Check sheet for the modelled part. Datum: model origin and axes. Units: mm. Face numbers are marked on the shaded views. A direction names the side the tool comes from. Give positions to 0.01 mm unless a question says otherwise; leave off trailing zeros. Order: outer loops, then holes, each group sorted by start corner. A loop starts at its lowest first (then second) coordinate and runs counter-clockwise, first axis right, second up.
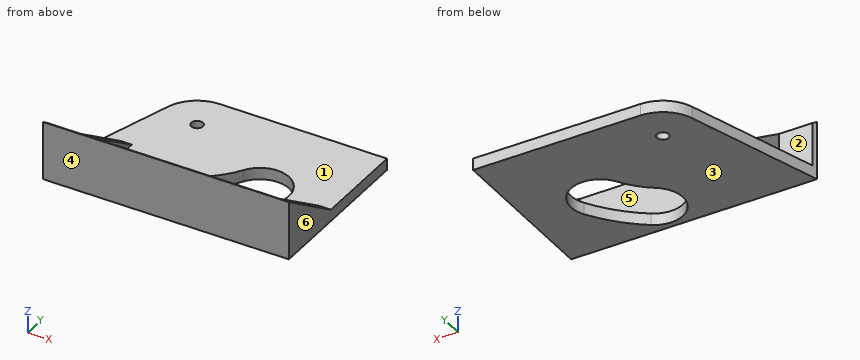
```python
from build123d import *

# Parameters (mm, degrees)
SKETCH1_W           = 120
SKETCH1_H           = 100
BOSS_EXTRUDE1_DEPTH = 5
SKETCH2_R           = 2.5
CUT_EXTRUDE1_DEPTH  = 6
SKETCH3_W           = 120
SKETCH3_H           = 2
BOSS_EXTRUDE2_DEPTH = 20
CUT_EXTRUDE2_DEPTH  = 26
CUT_EXTRUDE3_DEPTH  = 26
SKETCH6_W           = 5
SKETCH6_H           = 30
BOSS_EXTRUDE3_DEPTH = 20
CUT_EXTRUDE4_DEPTH  = 106
SKETCH10_W          = 27.884556649
SKETCH10_H          = 70
CUT_EXTRUDE5_DEPTH  = 106


with BuildPart() as part:
    # Sketch1 → Boss-Extrude1 (new body)
    with BuildSketch(Plane.XY):
        with Locations((60, 50)):
            Rectangle(SKETCH1_W, SKETCH1_H)
    boss_extrude1 = extrude(amount=BOSS_EXTRUDE1_DEPTH)

    # Sketch2 → Cut-Extrude1 (cut, through all)
    with BuildSketch(Plane.XY.offset(5)):
        with Locations((48.561388608, 53.909722104)):
            Circle(SKETCH2_R)
        with BuildLine():
            ThreePointArc((82.975974789, 4.760599446), (92.719162031, 13.288409394), (100.405906554, 23.707967867))
            ThreePointArc((100.405906554, 23.707967867), (95.896997447, 40.800941239), (78.804024076, 36.292032133))
            ThreePointArc((78.804024076, 36.292032133), (74.320089771, 30.213956356), (68.63656388, 25.239400554))
            ThreePointArc((68.63656388, 25.239400554), (65.566868781, 7.830294546), (82.975974789, 4.760599446))
        make_face()
    cut_extrude1 = extrude(amount=-CUT_EXTRUDE1_DEPTH, mode=Mode.SUBTRACT)

    # Sketch3 → Boss-Extrude2 (add)
    with BuildSketch(Plane(origin=(0, 0, 0), x_dir=(-1, 0, 0), z_dir=(0, 0, -1))):
        with Locations((-60, 1)):
            Rectangle(SKETCH3_W, SKETCH3_H)
    boss_extrude2 = extrude(amount=BOSS_EXTRUDE2_DEPTH)

    # Sketch4 → Cut-Extrude2 (cut, through all)
    with BuildSketch(Plane.XY.offset(5)):
        with BuildLine():
            ThreePointArc((66.494283868, 35.596794606), (72.644903394, 39.60143936), (75.487572744, 46.368013909))
            ThreePointArc((75.487572744, 46.368013909), (73.248961533, 49.104548186), (70.512427256, 46.865936976))
            ThreePointArc((70.512427256, 46.865936976), (68.806825647, 42.805992246), (65.116453931, 40.403205394))
            ThreePointArc((65.116453931, 40.403205394), (63.402163505, 37.311085032), (66.494283868, 35.596794606))
        make_face()
    extrude(amount=-CUT_EXTRUDE2_DEPTH, mode=Mode.SUBTRACT)

    # Sketch5 → Cut-Extrude3 (cut, through all)
    with BuildSketch(Plane.XY.offset(5)):
        with BuildLine():
            Line((120, 70), (48.561388608, 70))
            ThreePointArc((48.561388608, 70), (39.016134462, 66.862913451), (33.192915272, 58.674915711))
            Line((33.192915272, 58.674915711), (15, 0))
            Line((15, 0), (0, 0))
            Line((0, 0), (0, 100))
            Line((0, 100), (120, 100))
            Line((120, 100), (120, 70))
        make_face()
    cut_extrude3 = extrude(amount=-CUT_EXTRUDE3_DEPTH, mode=Mode.SUBTRACT)

    # Sketch6 → Boss-Extrude3 (add, through all)
    with BuildSketch(Plane(origin=(0, 0, 0), x_dir=(-1, 0, 0), z_dir=(0, 0, -1))):
        with Locations((-117.5, 15)):
            Rectangle(SKETCH6_W, SKETCH6_H)
        with Locations((-32.5, 15)):
            Rectangle(SKETCH6_W, SKETCH6_H)
    boss_extrude3 = extrude(amount=BOSS_EXTRUDE3_DEPTH)

    # Sketch9 → Cut-Extrude4 (cut, through all)
    with BuildSketch(Plane(origin=(120, 0, 0), x_dir=(0, 0, -1), z_dir=(1, 0, 0))):
        Polygon((0, 30), (20, 0), (20, 30), align=None)
    cut_extrude4 = extrude(amount=-CUT_EXTRUDE4_DEPTH, mode=Mode.SUBTRACT)

    # Mirror1: Boss-Extrude1, Cut-Extrude1, Boss-Extrude2, Cut-Extrude3, Boss-Extrude3, Cut-Extrude4 across plane
    add(boss_extrude1.mirror(Plane(origin=(0, 0, 5), x_dir=(1, 0, 0), z_dir=(0, 0, -1))))
    add(cut_extrude1.mirror(Plane(origin=(0, 0, 5), x_dir=(1, 0, 0), z_dir=(0, 0, -1))), mode=Mode.SUBTRACT)
    add(boss_extrude2.mirror(Plane(origin=(0, 0, 5), x_dir=(1, 0, 0), z_dir=(0, 0, -1))))
    add(cut_extrude3.mirror(Plane(origin=(0, 0, 5), x_dir=(1, 0, 0), z_dir=(0, 0, -1))), mode=Mode.SUBTRACT)
    add(boss_extrude3.mirror(Plane(origin=(0, 0, 5), x_dir=(1, 0, 0), z_dir=(0, 0, -1))))
    add(cut_extrude4.mirror(Plane(origin=(0, 0, 5), x_dir=(1, 0, 0), z_dir=(0, 0, -1))), mode=Mode.SUBTRACT)

    # Sketch10 → Cut-Extrude5 (cut, through all)
    with BuildSketch(Plane(origin=(120, 0, 0), x_dir=(0, 0, -1), z_dir=(1, 0, 0))):
        with Locations((8.942278325, 35)):
            Rectangle(SKETCH10_W, SKETCH10_H)
    extrude(amount=-CUT_EXTRUDE5_DEPTH, mode=Mode.SUBTRACT)


solid = part.part
```
(1) Release check for a two-part mould opening along X. For the marked faces 4, 5 and 6 record: released by +X, released by -X, zero draft, split by the parting line, or undercut.
Response values:
face 4: zero draft
face 5: undercut
face 6: released by +X
(2) Material ranges on L1, parallel to Z at x = 20.5, y = 15.5; L2, parallel to Y at x = 25, z = 18; L3, parallel to X at y = 12.5, z = 19, recorded low to high.
Response values:
L1: z = 5 to 10
L2: y = 0 to 2
L3: x = 30 to 35, 115 to 120
(3) Cross-section at D-D on x = 57. Enter the section's corners in (y, z), then the cut area to 3 significant figures.
Response values:
outline: (0, 5) - (70, 5) - (70, 10) - (2, 10) - (2, 28.67) - (0, 30) - close
area: 389 mm2
(4) Cross-section at B-B on z = 14. Enter the section's corners in (x, y).
Response values:
outline: (15, 0) - (120, 0) - (120, 24) - (115, 24) - (115, 2) - (35, 2) - (35, 24) - (30, 24) - (30, 2) - (15.62, 2) - close
(5) Gauge pin test, flat ends, axial feed: pin 1 Ø15 at (y, z) = (16, 22.5) entering from +X; pin 2 Ø15 at (y, z) = (13.5, 20) entering from -X; pin 3 Ø8 at (x, y) = (52.5, 39.5) entering from +Z. Record the tip position at first contact, or that the pin passes through.
Response values:
pin 1: stops at x = 120
pin 2: stops at x = 30
pin 3: stops at z = 10
(6) Cross-section at A-A on y = 14.5. Enter the section's corners in (x, z).
Response values:
outline: (19.5, 5) - (63.32, 5) - (63.32, 10) - (35, 10) - (35, 20.33) - (30, 20.33) - (30, 10) - (19.5, 10) - close; (93.8, 5) - (120, 5) - (120, 20.33) - (115, 20.33) - (115, 10) - (93.8, 10) - close
(7) Set-up check for the marked faces 1, 2 and 3: record each of +Z, -Z, +X, -X, +Y, -Y from which the full face is reachable in a straight line by a thin tool's end or side.
Response values:
face 1: +Z, +Y
face 2: +Z, -X, +Y
face 3: -Z, +X, -X, +Y, -Y
(8) Cross-section at C-C on x = 72. Enter the section's corners in (y, z).
Response values:
outline: (0, 5) - (3.09, 5) - (3.09, 10) - (2, 10) - (2, 28.67) - (0, 30) - close; (27.92, 5) - (70, 5) - (70, 10) - (27.92, 10) - close
